from build123d import *

# Parameters (mm, degrees)
CHAMFER1_SIZE = 0.5
FILLET1_R     = 0.3


with BuildPart() as part:
    # Sketch1 → Revolve1 (revolve)
    with BuildSketch(Plane.XY):
        Polygon((-608.6, 54.57), (-636.6, 54.57), (-636.6, 51.57), (-70.6, 51.57), (-70.6, 54.57), (-93.6, 54.57), (-93.6, 57.57), (-608.6, 57.57), align=None)
    revolve(axis=Axis((-24.960657764, 51.57, 0), (-1, 0, 0)))

    # Chamfer1
    chamfer1_edges = [part.edges().sort_by_distance(p)[0] for p in [
        (-70.6, 48.57, 0),
        (-636.6, 48.57, 0),
    ]]
    chamfer(chamfer1_edges, length=CHAMFER1_SIZE)

    # Fillet1
    fillet1_edges = [part.edges().sort_by_distance(p)[0] for p in [
        (-93.6, 48.57, 0),
        (-608.6, 48.57, 0),
    ]]
    fillet(fillet1_edges, radius=FILLET1_R)


solid = part.part
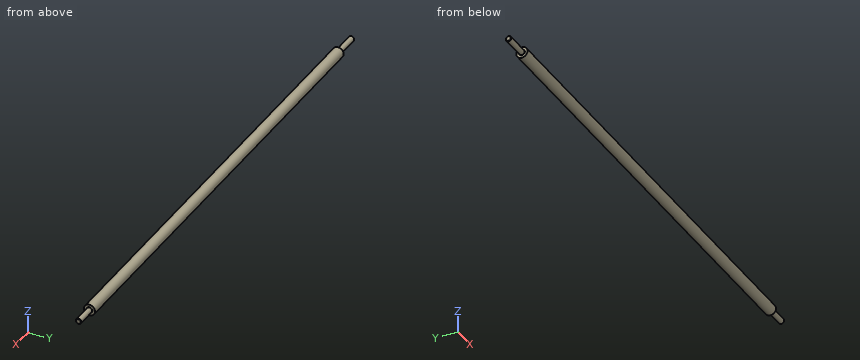
The listing builds one solid part. Answer for the finished solid, in the listing's coordinates (mm). Coordinates: 2 decimals unless noted, no trailing zeros. Loops run counter-clockwise (first coordinate to the right, second up) from the corner with the lowest first, then second, coordinate; pieces in that order, holes last.
1) Find the intervals of material crossed by L1, parallel to Z at x = -273, y = 52; L2, parallel to Z at x = -350, y = 50.5; L3, parallel to X at y = 56, z = 3.25, in increasing order.
2) Find section C-C on x = -463.5. Write down the section's boundary in (y, z), then the cut area to 3 significant figures.
3) Flat-ended cylindrical pins translate along their axes: pin 1 Ø2 at (x, z) = (-261.5, 4) entering from +Y; pin 2 Ø6 at (x, y) = (-343, 56) entering from -Z; pin 3 Ø1 at (y, z) = (56, 0.5) entering from -X. Find the tip coordinate at first contact, or state that the pin passes through.
4) Find section A-A on z = 0. Write down the section's boundary in (x, y).
5) Find section B-B on y = 51.57. Write down the section's boundary in (x, z), then the cut area to 3 significant figures.
Values:
1. L1: z = -5.98 to 5.98
1. L2: z = -5.9 to 5.9
1. L3: x = -608.6 to -93.6
2. outline: circle Ø12 at (51.57, 0)
2. area: 113 mm2
3. pin 1: stops at y = 56.77
3. pin 2: stops at z = -5.83
3. pin 3: stops at x = -608.6
4. outline: (-636.6, 49.07) - (-636.1, 48.57) - (-608.9, 48.57) arc R0.3 cw to (-608.6, 48.27) - (-608.6, 45.57) - (-93.6, 45.57) - (-93.6, 48.27) arc R0.3 cw to (-93.3, 48.57) - (-71.1, 48.57) - (-70.6, 49.07) - (-70.6, 54.07) - (-71.1, 54.57) - (-93.3, 54.57) arc R0.3 cw to (-93.6, 54.87) - (-93.6, 57.57) - (-608.6, 57.57) - (-608.6, 54.87) arc R0.3 cw to (-608.9, 54.57) - (-636.1, 54.57) - (-636.6, 54.07) - close
5. outline: (-636.6, -2.5) - (-636.1, -3) - (-608.9, -3) arc R0.3 cw to (-608.6, -3.3) - (-608.6, -6) - (-93.6, -6) - (-93.6, -3.3) arc R0.3 cw to (-93.3, -3) - (-71.1, -3) - (-70.6, -2.5) - (-70.6, 2.5) - (-71.1, 3) - (-93.3, 3) arc R0.3 cw to (-93.6, 3.3) - (-93.6, 6) - (-608.6, 6) - (-608.6, 3.3) arc R0.3 cw to (-608.9, 3) - (-636.1, 3) - (-636.6, 2.5) - close
5. area: 6,490 mm2
